from build123d import *

# Parameters (mm, degrees)
SKETCH123_W      = 18
SKETCH123_H      = 13
EXTRUDE112_DEPTH = 5


with BuildPart() as extrude112:
    # Sketch123 → Extrude112 (new body)
    with BuildSketch(Plane.YZ.offset(50)):
        with Locations((51, -18.5)):
            Rectangle(SKETCH123_W, SKETCH123_H)
    extrude(amount=-EXTRUDE112_DEPTH)


with BuildPart() as cut019:
    # Sweep: sweep along a path in Sketch090
    with BuildLine(Plane(origin=(0, 0, -28), x_dir=(1, 0, 0), z_dir=(0, 0, -1))) as sweep_path:
        Line((16.5, -35.5), (47.5, -35.5))
        Line((47.5, -35.5), (47.5, -66.5))
        Line((47.5, -66.5), (16.5, -66.5))
        Line((16.5, -66.5), (16.5, -35.5))
    # Sketch089 → Sweep (sweep)
    with BuildSketch(Plane.XZ.offset(-34)):
        Polygon((16, -14.5), (16.5, -14.5), (16.5, -30), (14.5, -30), (14.5, -15.5), (16, -15.5), align=None)
    sweep(path=sweep_path.line, transition=Transition.RIGHT)

    # Cut019: cut Extrude112
    add(extrude112.part, mode=Mode.SUBTRACT)


solid = cut019.part
Check sheet for the modelled part. Datum: model origin and axes. Units: mm. A direction names the side the tool comes from. Give positions to 0.01 mm unless a question says otherwise; leave off trailing zeros. Loops run counter-clockwise (first coordinate to the right, second up) from the corner with the lowest first, then second, coordinate; pieces in that order, holes last. Notation, with made-up numbers: M 15,-15 L 21,-15 A20 cw 21,13 Z; hole C -17.5,80.25 d8. An arc over 180 degrees is marked long. Answer as a JSON object with one key per item and string values. Group by question number.
Q1. Material ranges on line 1 along Y through (x, z) = (47, -24); line 2 along X through (y, z) = (37, -25.25); line 3 along Y through (x, z) = (48, -22), recorded low to high. Write a range as [from, to].
Q2. Cross-section at C-C on y = 62.5. Record the cut outline in (x, z).
Q3. Access from +Z, -Z, +X, -X, +Y, -Y to the whole of each face (thin tool, end or side, straight path). Record for faces 1 (the flat face through (32, 35.5, -22)), 2 (the flat face through (49, 42, -20)), 3 (the flat face through (32, 35, -15)), 4 (the flat face through (48, 64, -15)).
Q4. Go/stop test with flat-tipped pins: P1, Ø0.8, axis at y = 37.5, z = -15, coming from the +X side; P2, Ø1, axis at y = 49, z = -23, coming from the +X side; P3, Ø1.6, axis at x = 49, y = 50.5, coming from the +Z side; P4, Ø12, axis at x = 39.5, y = 44, coming from the -Z side. Record where each tip stops, or that it passes through.
Q5. Cross-section at D-D on z = -21.5. Record the cut outline in (x, y), then the cut area to 3 significant figures.
Q6. Cross-section at A-A on z = -26. Record the cut outline in (x, y).
Q7. Release check for a two-part mould opening along X. For faces 5 (the flat face through (32, 66.5, -22)), 6 (the flat face through (35, 35, -30)), 7 (the flat face through (16.5, 51, -22)), 8 (the flat face through (48, 39, -15)) record: released by +X, released by -X, zero draft, split by the parting line, or undercut.
Q8. Cross-section at B-B on x = 30.5. Record the cut outline in (y, z).
Evaluation:
{
 "1": {"line 1": "y = [33.5, 35.5], [66.5, 68.5]", "line 2": "x = [14.5, 16.5], [47.5, 49.5]", "line 3": "y = [33.5, 42], [60, 68.5]"},
 "2": {"outline": "M 14.5,-30 L 16.5,-30 L 16.5,-14.5 L 16,-14.5 L 16,-15.5 L 14.5,-15.5 Z; M 47.5,-30 L 49.5,-30 L 49.5,-15.5 L 48,-15.5 L 48,-14.5 L 47.5,-14.5 Z"},
 "3": {"face 1": "+Z, -Z", "face 2": "+Z, +X", "face 3": "+Z, +X, -X, -Y", "face 4": "+Z, +X, +Y, -Y"},
 "4": {"P1": "stops at x = 48", "P2": "stops at x = 16.5", "P3": "stops at z = -25", "P4": "passes through"},
 "5": {"outline": "M 14.5,33.5 L 49.5,33.5 L 49.5,42 L 47.5,42 L 47.5,35.5 L 16.5,35.5 L 16.5,66.5 L 47.5,66.5 L 47.5,60 L 49.5,60 L 49.5,68.5 L 14.5,68.5 Z", "area": "228 mm2"},
 "6": {"outline": "M 14.5,33.5 L 49.5,33.5 L 49.5,68.5 L 14.5,68.5 Z; hole M 16.5,35.5 L 47.5,35.5 L 47.5,66.5 L 16.5,66.5 Z"},
 "7": {"face 5": "undercut", "face 6": "zero draft", "face 7": "undercut", "face 8": "released by +X"},
 "8": {"outline": "M 33.5,-30 L 35.5,-30 L 35.5,-14.5 L 35,-14.5 L 35,-15.5 L 33.5,-15.5 Z; M 66.5,-30 L 68.5,-30 L 68.5,-15.5 L 67,-15.5 L 67,-14.5 L 66.5,-14.5 Z"}
}
